Model file for the job. Use its own axes, mm. Face numbers are marked on the shaded views. A direction names the side the tool comes from. Round coordinates to 2 decimals unless told otherwise and drop trailing zeros. Write each loop counter-clockwise with the first axis right and the second up, starting at its lowest first coordinate (ties: lowest second). Pieces come first, ordered by that corner, then holes. Notation, with made-up numbers: (-8.75, 67.5) - (37.25, 67.5) arc R17 ccw to (37.25, 73.5) - close; hole circle Ø11 at (21.5, 40.5). An arc over 180 degrees is marked (long way). Answer as a JSON object with one key per item and string values. Group by question number.
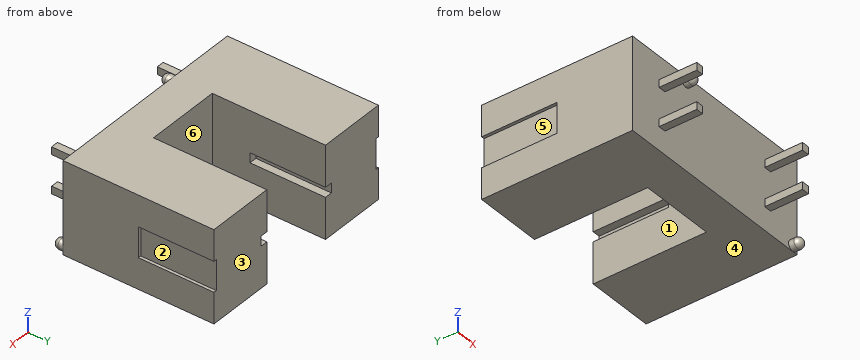
from build123d import *

# Parameters (mm, degrees)
EXTRUDE1_DEPTH           = 3.05
EXTRUDE1_DEPTH_BACK      = 3.05
SKETCH2_W                = 0.5
SKETCH2_H                = 2.5
EXTRUDE_THIN1_DEPTH      = 0.25
EXTRUDE_THIN1_DEPTH_BACK = 0.25
SKETCH2_3_W              = 0.5
SKETCH2_3_H              = 2.5
EXTRUDE_THIN2_DEPTH      = 0.25
EXTRUDE_THIN2_DEPTH_BACK = 0.25
SKETCH3_W                = 0.5
SKETCH3_H                = 2.5
EXTRUDE_THIN3_DEPTH      = 0.25
EXTRUDE_THIN3_DEPTH_BACK = 0.25
SKETCH3_3_W              = 0.5
SKETCH3_3_H              = 2.5
EXTRUDE_THIN4_DEPTH      = 0.25
EXTRUDE_THIN4_DEPTH_BACK = 0.25
SKETCH4_R                = 0.35
EXTRUDE2_DEPTH           = 0.7
FILLET1_R                = 0.35
SKETCH5_W                = 2
SKETCH5_H                = 5
CUT_EXTRUDE1_DEPTH       = 0.2
SKETCH6_W                = 2
SKETCH6_H                = 5
CUT_EXTRUDE2_DEPTH       = 0.2
SKETCH7_W                = 0.65
SKETCH7_H                = 5.045356776
CUT_EXTRUDE3_DEPTH       = 0.5
SKETCH8_W                = 0.65
SKETCH8_H                = 5.045356776
CUT_EXTRUDE4_DEPTH       = 0.5


with BuildPart() as part:
    # Sketch1 → Extrude1 (new body, two sides)
    with BuildSketch(Plane.XY) as extrude1_sk:
        Polygon((2.5, 10), (7, 10), (7, 0), (-7, 0), (-7, 10), (-2.5, 10), (-2.5, 2.5), (2.5, 2.5), align=None)
    extrude(amount=EXTRUDE1_DEPTH)
    extrude(extrude1_sk.sketch, amount=-EXTRUDE1_DEPTH_BACK)

    # Sketch2 → Extrude-Thin1 (add, two sides)
    with BuildSketch(Plane(origin=(4.5, 0, 0), x_dir=(0, 0, -1), z_dir=(1, 0, 0))) as extrude_thin1_sk:
        with Locations((1.27, -1.25)):
            Rectangle(SKETCH2_W, SKETCH2_H)
    extrude(amount=EXTRUDE_THIN1_DEPTH)
    extrude(extrude_thin1_sk.sketch, amount=-EXTRUDE_THIN1_DEPTH_BACK)

    # Sketch2_3 → Extrude-Thin2 (add, two sides)
    with BuildSketch(Plane(origin=(4.5, 0, 0), x_dir=(0, 0, -1), z_dir=(1, 0, 0))) as extrude_thin2_sk:
        with Locations((1.27, -1.25)):
            Rectangle(SKETCH2_3_W, SKETCH2_3_H)
        with Locations((-1.27, -1.25)):
            Rectangle(SKETCH2_3_W, SKETCH2_3_H)
    extrude(amount=EXTRUDE_THIN2_DEPTH)
    extrude(extrude_thin2_sk.sketch, amount=-EXTRUDE_THIN2_DEPTH_BACK)

    # Sketch3 → Extrude-Thin3 (add, two sides)
    with BuildSketch(Plane(origin=(-4.5, 0, 0), x_dir=(0, 0, -1), z_dir=(1, 0, 0))) as extrude_thin3_sk:
        with Locations((1.27, -1.25)):
            Rectangle(SKETCH3_W, SKETCH3_H)
    extrude(amount=EXTRUDE_THIN3_DEPTH)
    extrude(extrude_thin3_sk.sketch, amount=-EXTRUDE_THIN3_DEPTH_BACK)

    # Sketch3_3 → Extrude-Thin4 (add, two sides)
    with BuildSketch(Plane(origin=(-4.5, 0, 0), x_dir=(0, 0, -1), z_dir=(1, 0, 0))) as extrude_thin4_sk:
        with Locations((-1.27, -1.25)):
            Rectangle(SKETCH3_3_W, SKETCH3_3_H)
        with Locations((1.27, -1.25)):
            Rectangle(SKETCH3_3_W, SKETCH3_3_H)
    extrude(amount=EXTRUDE_THIN4_DEPTH)
    extrude(extrude_thin4_sk.sketch, amount=-EXTRUDE_THIN4_DEPTH_BACK)

    # Sketch4 → Extrude2 (add)
    with BuildSketch(Plane(origin=(0, 0, 0), x_dir=(1, 0, 0), z_dir=(0, 1, 0))):
        with Locations((-2.45, -2.685779489)):
            Circle(SKETCH4_R)
        with Locations((6.630550891, 2.686987207)):
            Circle(SKETCH4_R)
    extrude(amount=-EXTRUDE2_DEPTH)

    # Fillet1
    fillet1_edges = [part.edges().sort_by_distance(p)[0] for p in [
        (-2.8, -0.7, 2.685779489),
        (6.280550891, -0.7, -2.686987207),
    ]]
    fillet(fillet1_edges, radius=FILLET1_R)

    # Sketch5 → Cut-Extrude1 (cut)
    with BuildSketch(Plane(origin=(7, 0, 0), x_dir=(0, 0, -1), z_dir=(1, 0, 0))):
        with Locations((0, 7.5)):
            Rectangle(SKETCH5_W, SKETCH5_H)
    extrude(amount=-CUT_EXTRUDE1_DEPTH, mode=Mode.SUBTRACT)

    # Sketch6 → Cut-Extrude2 (cut)
    with BuildSketch(Plane.ZY.offset(7)):
        with Locations((0, 7.5)):
            Rectangle(SKETCH6_W, SKETCH6_H)
    extrude(amount=-CUT_EXTRUDE2_DEPTH, mode=Mode.SUBTRACT)

    # Sketch7 → Cut-Extrude3 (cut)
    with BuildSketch(Plane.ZY.offset(-2.5)):
        with Locations((0, 7.522678388)):
            Rectangle(SKETCH7_W, SKETCH7_H)
    extrude(amount=-CUT_EXTRUDE3_DEPTH, mode=Mode.SUBTRACT)

    # Sketch8 → Cut-Extrude4 (cut)
    with BuildSketch(Plane(origin=(-2.5, 0, 0), x_dir=(0, 0, -1), z_dir=(1, 0, 0))):
        with Locations((0, 7.522678388)):
            Rectangle(SKETCH8_W, SKETCH8_H)
    extrude(amount=-CUT_EXTRUDE4_DEPTH, mode=Mode.SUBTRACT)


solid = part.part
(1) Drill centre lines: line 1 (X direction, y = 8.25, z = 1.5); line 2 (Y direction, x = -0.5, z = -1.75); line 3 (X direction, y = 7.5, z = 0). Where is each one in solid material? Low to high. Write a range as from..to.
(2) Slice it at B-B (z = 2). Write the cut outline in (x, y), then the cut area to 4 significant figures.
(3) Slice it at A-A (y = -1.25). Write the cut outline in (x, z), then the cut area to 3 significant figures.
(4) Flat gauge pins, fed straight in: pin 1 (3 mm diameter, centred on x = 5.5, z = -1, fed in from -Y); pin 2 (0.6 mm diameter, centred on y = -1, z = 1, fed in from +X). Where does each tip first touch, or does it go through?
(5) Slice it at D-D (x = -5). Write the cut outline in (y, z).
(6) Slice it at C-C (y = 7). Write the cut outline in (x, z) (3 decimals).
(7) Pull direction Z, two halves, no side cores. Call the marked faces 4, 5 and 6: pulls with the +Z half, pulls with the -Z half, needs draft (parallel to the pull), parting line crosses it, or undercut.
(8) 3-axis set-ups, long thin cutter, end or side, ignore diameter. For the marked faces 1, 2 and 3: which of +Z, -Z, +X, -X, +Y, -Y reach the whole face in a straight line?
Answer:
{
 "1": {"line 1": "-7..-2.5, 2.5..7", "line 2": "0..2.5", "line 3": "-6.8..-3, 3..6.8"},
 "2": {"outline": "(-7, 0) - (7, 0) - (7, 10) - (2.5, 10) - (2.5, 2.5) - (-2.5, 2.5) - (-2.5, 10) - (-7, 10) - close", "area": "102.5 mm²"},
 "3": {"outline": "(-4.75, -1.52) - (-4.25, -1.52) - (-4.25, -1.02) - (-4.75, -1.02) - close; (-4.75, 1.02) - (-4.25, 1.02) - (-4.25, 1.52) - (-4.75, 1.52) - close; (4.25, -1.52) - (4.75, -1.52) - (4.75, -1.02) - (4.25, -1.02) - close; (4.25, 1.02) - (4.75, 1.02) - (4.75, 1.52) - (4.25, 1.52) - close", "area": "1.00 mm²"},
 "4": {"pin 1": "y = -2.5", "pin 2": "x = 4.75"},
 "5": {"outline": "(0, -3.05) - (10, -3.05) - (10, 3.05) - (0, 3.05) - close"},
 "6": {"outline": "(-7, -3.05) - (-2.5, -3.05) - (-2.5, -0.325) - (-3, -0.325) - (-3, 0.325) - (-2.5, 0.325) - (-2.5, 3.05) - (-7, 3.05) - (-7, 1) - (-6.8, 1) - (-6.8, -1) - (-7, -1) - close; (2.5, -3.05) - (7, -3.05) - (7, -1) - (6.8, -1) - (6.8, 1) - (7, 1) - (7, 3.05) - (2.5, 3.05) - (2.5, 0.325) - (3, 0.325) - (3, -0.325) - (2.5, -0.325) - close"},
 "7": {"face 4": "pulls with the -Z half", "face 5": "undercut", "face 6": "needs draft"},
 "8": {"face 1": "+Z, -Z, +Y", "face 2": "+X, +Y", "face 3": "+Z, -Z, +X, -X, +Y"}
}
